from build123d import *

# Parameters (mm, degrees)
SKETCH1_R      = 1.65
EXTRUDE1_DEPTH = 4
SKETCH3_R      = 2.25
EXTRUDE3_DEPTH = 4


with BuildPart() as part:
    # Sketch1 → Extrude1 (new body)
    with BuildSketch(Plane(origin=(0, 0, 0), x_dir=(1, 0, 0), z_dir=(0, 1, 0))):
        Polygon((-80, 10), (-80, -75), (80, -75), (80, 10), (72, 10), (72, 75), (45, 75), (45, -3), (63, -3), (63, -63), (-63, -63), (-63, -3), (-45, -3), (-45, 75), (-72, 75), (-72, 10), align=None)
        with Locations((-67, -63)):
            Circle(SKETCH1_R, mode=Mode.SUBTRACT)
        with Locations((67, -63)):
            Circle(SKETCH1_R, mode=Mode.SUBTRACT)
        with Locations((-67, 67)):
            Circle(SKETCH1_R, mode=Mode.SUBTRACT)
        with Locations((58, 65)):
            Circle(SKETCH1_R, mode=Mode.SUBTRACT)
    extrude(amount=EXTRUDE1_DEPTH)

    # Sketch3 → Extrude3 (cut)
    with BuildSketch(Plane(origin=(0, 4, 0), x_dir=(1, 0, 0), z_dir=(0, 1, 0))):
        with Locations((52.5, -67.259837658)):
            Circle(SKETCH3_R)
        with Locations((-52.5, -67.259837658)):
            Circle(SKETCH3_R)
        with Locations((52.5, 37.740162342)):
            Circle(SKETCH3_R)
        with Locations((-52.5, 37.740162342)):
            Circle(SKETCH3_R)
    extrude(amount=-EXTRUDE3_DEPTH, mode=Mode.SUBTRACT)


solid = part.part
Geometry: final body of the model. Coordinates: model frame, mm. A direction names the side the tool comes from. Round coordinates to 2 decimals unless told otherwise and drop trailing zeros. Order: outer loops, then holes, each group sorted by start corner. A loop starts at its lowest first (then second) coordinate and runs counter-clockwise, first axis right, second up. Notation, with made-up numbers: (13.5, -33) - (28.5, -33) arc R6 ccw to (28.5, -28) - close; hole circle Ø3 at (54.25, -2.5). An arc over 180 degrees is marked (long way). Write each question's results on one line, items separated by ' | '.
Item 1: Section D-D, the plane z = -23. Return the cut outline in (x, y), and give its area (3 significant figures).
Completed:
outline: (-72, 0) - (-45, 0) - (-45, 4) - (-72, 4) - close; (45, 0) - (72, 0) - (72, 4) - (45, 4) - close | area: 216 mm^2
Item 2: Section A-A, the plane z = -8. Return the cut outline in (x, y).
Completed:
outline: (-80, 0) - (-45, 0) - (-45, 4) - (-80, 4) - close; (45, 0) - (80, 0) - (80, 4) - (45, 4) - close
Item 3: Material intervals for line 1 along Z through (x, y) = (-52.5, 3.1); line 2 along Z through (x, y) = (67, 2.5); line 3 along X through (y, z) = (3, -7.5), sorted ascending. Write a range as [from, to].
Completed:
line 1: [-75, -39.99], [-35.49, 3], [63, 65.01], [69.51, 75] | line 2: [-75, 61.35], [64.65, 75] | line 3: [-80, -45], [45, 80]
Item 4: Mould query, pull axis Z, two halves, no side actions, for faces 1 (the flat face through (-76, 2, -10)), 2 (the flat face through (-72, 2, -43)), 3 (the cylindrical face through (-67.4, 2, -65.4)). Classes: pulls with the +Z half, pulls with the -Z half, needs draft (parallel to the pull), parting line crosses it, or undercut.
Completed:
face 1: pulls with the -Z half | face 2: needs draft | face 3: undercut
Item 5: Section B-B, the plane x = 52.5. Return the cut outline in (y, z).
Completed:
outline: (0, -75) - (4, -75) - (4, -39.99) - (0, -39.99) - close; (0, -35.49) - (4, -35.49) - (4, 3) - (0, 3) - close; (0, 63) - (4, 63) - (4, 65.01) - (0, 65.01) - close; (0, 69.51) - (4, 69.51) - (4, 75) - (0, 75) - close
Item 6: Section C-C, the plane y = 1.05. State how many separate pieces and enclosed holes the cut face has, and give its area (3 significant figures).
Completed:
separate pieces: 1 | enclosed holes: 8 | area: 8,280 mm^2
Item 7: Reachability of faces 4 (the flat face through (54, 2, 3)), 5 (the flat face through (52, 4, -1)), 6 (the flat face through (76, 2, -10)), 7 (the flat face through (45, 2, -37)) from +Z, -Z, +X, -X, +Y, -Y: full face, straight path, thin tool, end or side. Return the list, or none.
Completed:
face 4: +Y, -Y | face 5: +Z, -Z, +X, -X, +Y | face 6: -Z, +X, +Y, -Y | face 7: -Z, +Y, -Y
Item 8: First-contact query: pin 1 Ø2 at (y, z) = (2, -32.5) entering from +X; pin 2 Ø1.2 at (y, z) = (2, -41.5) entering from -X. Flat tips, straight axial feed; report the tip coordinate or a pass-through.
Completed:
pin 1: x = 72 | pin 2: x = -72
